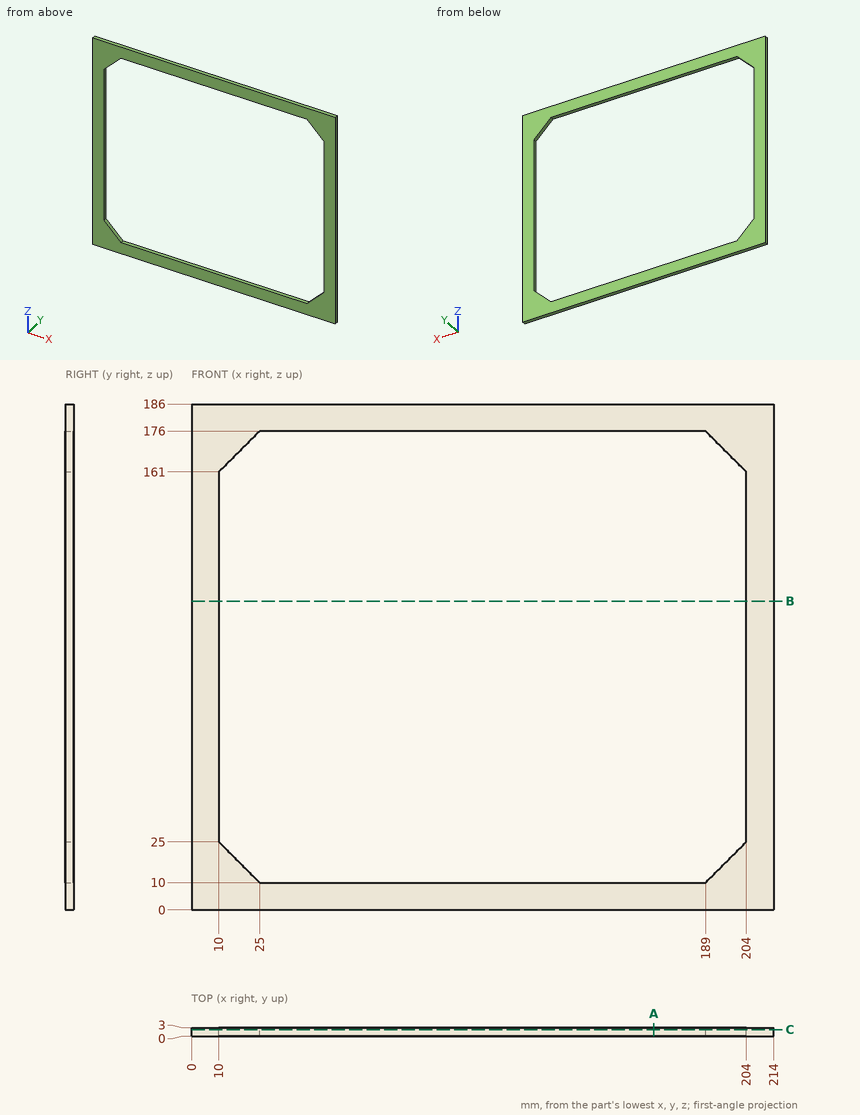
Study the drawing (mm; zero at the part's minimum x, y, z) and answer. Round coordinates to 2 decimals unless told otherwise and drop trailing zeros. Write each loop counter-clockwise with the first axis right and the second up, starting at its lowest first coordinate (ties: lowest second). Pieces come first, ordered by that corner, then holes. Notation, with made-up numbers: (59, 15.25) -> (65, 15.25) arc R13 cw to (65, 21.25) -> close; hole circle Ø2 at (61.25, 0.25). An arc over 180 degrees is marked (long way). Write each question's results on one line, items separated by ' | '.
Item 1: Find the intervals of material crossed by line 1 along X through (y, z) = (1.9, 120); line 2 along Z through (x, y) = (175.5, 2.6); line 3 along Z through (x, y) = (199, 2.8), in increasing order. Write a range as [from, to].
Result set:
line 1: [0, 10], [204, 214] | line 2: [0, 10], [176, 186] | line 3: [0, 20], [166, 186]
Item 2: A cutting plane is placed at C-C, the plane y = 2.35. Determine the outline of the cut face in (x, z).
Result set:
outline: (0, 0) -> (214, 0) -> (214, 186) -> (0, 186) -> close; hole (10, 25) -> (25, 10) -> (189, 10) -> (204, 25) -> (204, 161) -> (189, 176) -> (25, 176) -> (10, 161) -> close
Item 3: A cutting plane is placed at B-B, the plane z = 113.5. Determine the outline of the cut face in (x, y).
Result set:
outline: (0, 0) -> (10, 0) -> (10, 3) -> (0, 3) -> close; (204, 0) -> (214, 0) -> (214, 3) -> (204, 3) -> close
Item 4: A cutting plane is placed at A-A, the plane x = 170. Determine the outline of the cut face in (y, z).
Result set:
outline: (0, 0) -> (3, 0) -> (3, 10) -> (0, 10) -> close; (0, 176) -> (3, 176) -> (3, 186) -> (0, 186) -> close
